The model under review builds one solid part; all positions refer to its coordinate system, in mm. A direction names the side the tool comes from. Round coordinates to 2 decimals unless told otherwise and drop trailing zeros. Write each loop counter-clockwise with the first axis right and the second up, starting at its lowest first coordinate (ties: lowest second). Pieces come first, ordered by that corner, then holes. Notation, with made-up numbers: M 51,6.25 L 58,6.25 A5 cw 58,13.25 Z; hole C 44.5,87 d7. An arc over 180 degrees is marked long. One line per item, written item: value. Start each with the question number.
1) Tool access review of faces 4 (the face through (-10.8, 1.04, -1.04)), 5 (the face through (-9.568, -1.088, 0.616)), 6 (the face through (-3, -3, 0)): name each direction out of +Z, -Z, +X, -X, +Y, -Y from which nothing blocks a thin tool from reaching the whole face with its end or side.
2) Take a section at A-A, the plane x = 3.75. Write out the cut boundary in (y, z), and give its area (3 significant figures).
3) Take a section at C-C, the plane z = -3.75. Write out the cut boundary in (x, y).
4) Wall thickness on probe 1 along X at (y, z) = (2.75, 3); probe 2 along Z at (x, y) = (-8.5, -0.5); probe 3 along X at (y, z) = (0, -2.25): over which ranges is each line inside the solid? List them lowest first.
5) For P1, Ø0.7, axis at x = -9, y = 0.5, coming from the +Z side; P2, Ø1.5, axis at x = 3.5, z = 2.5, coming from the +Y side; P3, Ø0.7, axis at y = 0.5, z = -0.5, coming from the -X side; P4, Ø1.5, axis at x = -2.5, z = 4, coming from the +Y side, all flat-tipped, find the tip position at first contact; note any pin that passes through.
6) Take a section at D-D, the plane y = 4. Write out the cut boundary in (x, z).
7) Take a section at B-B, the plane y = 2.5. Write out the cut boundary in (x, z), and give its area (3 significant figures).
8) Mouldability with a two-part tool opening along Y and no side actions: class faces 1 (the face through (10.43, 0, 0)), 2 (the face through (-9.38, -1.08, -4.88)), 3 (the face through (-9.57, -1.08, -0.63)) as +Y half, -Y half, draft (parallel to the pull), parting line (faces both ways), or undercut.
Autodesk Inventor part; units mm, degrees
ref_plane "YZ Plane" through (0, 0, 0) normal (1, 0, 0) x (0, 1, 0)
ref_plane "XZ Plane" through (0, 0, 0) normal (0, 1, 0) x (-1, 0, 0)
ref_plane "XY Plane" through (0, 0, 0) normal (0, 0, 1) x (1, 0, 0)
sketch "Sketch_1" plane through (0, 0, 0) normal (0, 0, 1) x (1, 0, 0)
  line L0 (5, 0) -> (-10.8, 0)
  line L1 (-10.8, 0) -> (-10.8, 5)
  line L2 (-10.8, 5) -> (-8, 5)
  line L3 (-8, 5) -> (-8, 3)
  line L4 (-8, 3) -> (2, 3)
  line L5 (2, 3) -> (2, 2)
  line L6 (2, 2) -> (10, 2)
  line L7 (10, 2) -> (10.4295, 1.5705)
  line L8 (10.4295, 1.5705) -> (10.4295, 0)
  line L9 (10.4295, 0) -> (-10.8, 0)
  dimension "d6" = 2.8
  dimension "d7" = 10
  dimension "d8" = 8
revolve "Revolution1" add sketch "Sketch_1" angle 360 about axis through (5, 0, 0) along (1, 0, 0)
thread "Thread1"
sketch "Sketch_2" plane through (-10.8, 0, 0) normal (-1, 0, 0) x (0, 1, 0)
  line L0 (-1.4434, 0) -> (-0.7217, -1.25)
  line L1 (-0.7217, -1.25) -> (0.7217, -1.25)
  line L2 (0.7217, -1.25) -> (1.4434, 0)
  line L3 (1.4434, 0) -> (0.7217, 1.25)
  line L4 (0.7217, 1.25) -> (-0.7217, 1.25)
  line L5 (-0.7217, 1.25) -> (-1.4434, 0)
extrude "Extrusion1" cut sketch "Sketch_2" against normal blind 2.5
sketch "Sketch_3" plane through (0, 0, 0) normal (0, 0, 1) x (1, 0, 0)
  line L0 (-7.5783, 0) -> (-8.3, 0)
  line L1 (-8.3, 0) -> (-8.3, 1.25)
  line L2 (-8.3, 1.25) -> (-7.5783, 0)
  line L3 (-7.5783, 0) -> (-8.3, 0)
revolve "Revolution2" cut sketch "Sketch_3" angle 360 about axis through (-7.5783, 0, 0) along (1, 0, 0)
properties part number "DBB4-10-8" material "스테인리스스틸"
Checked values:
1. face 4: +Z, -Z, -X, +Y, -Y
1. face 5: -X
1. face 6: +X
2. outline: C 0,0 d4
2. area: 12.6 mm2
3. outline: M -10.8,-3.31 L -8,-3.31 L -8,3.31 L -10.8,3.31 Z
4. probe 1: x = -10.8 to -8
4. probe 2: z = -4.97 to -1.25, 1.25 to 4.97
4. probe 3: x = -10.8 to 2
5. P1: stops at z = 5
5. P2: stops at y = 0.97
5. P3: stops at x = -8.19
5. P4: passes through
6. outline: M -10.8,-3 L -8,-3 L -8,3 L -10.8,3 Z
7. outline: M -10.8,-4.33 L -8,-4.33 L -8,-1.66 L 2,-1.66 L 2,1.66 L -8,1.66 L -8,4.33 L -10.8,4.33 Z
7. area: 57.4 mm2
8. face 1: draft
8. face 2: parting line
8. face 3: undercut
